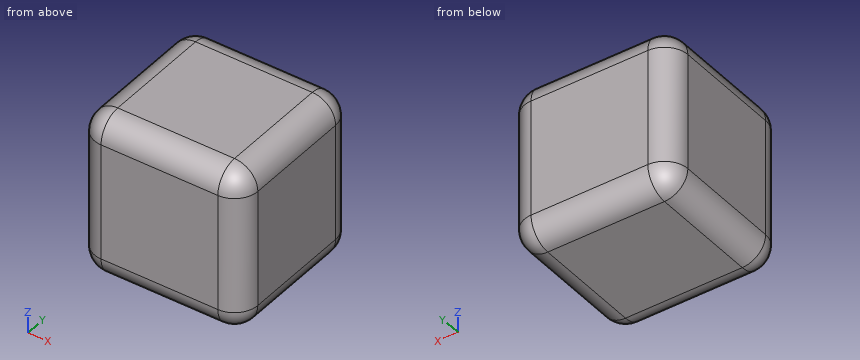
Autodesk Inventor part; units mm, degrees
ref_plane "YZ Plane" through (0, 0, 0) normal (1, 0, 0) x (0, 1, 0)
ref_plane "XZ Plane" through (0, 0, 0) normal (0, 1, 0) x (-1, 0, 0)
ref_plane "XY Plane" through (0, 0, 0) normal (0, 0, 1) x (1, 0, 0)
sketch "Эскиз1" plane through (0, 0, 0) normal (0, 1, 0) x (-1, 0, 0)
  line L0 (5.25, 5.25) -> (-5.25, 5.25)
  line L1 (-5.25, 5.25) -> (-5.25, -5.25)
  line L2 (-5.25, -5.25) -> (5.25, -5.25)
  line L3 (5.25, -5.25) -> (5.25, 5.25)
  line L4 (5.25, 0) -> (-5.25, 0) construction
  line L5 (0, 5.25) -> (0, -5.25) construction
  line L6 (3.5, -3.5) -> (-3.5, -3.5)
  line L7 (-3.5, -3.5) -> (-3.5, 3.5)
  line L8 (-3.5, 3.5) -> (3.5, 3.5)
  line L9 (3.5, 3.5) -> (3.5, -3.5)
  line L10 (0, -3.5) -> (0, 3.5) construction
  line L11 (3.5, 0) -> (-3.5, 0) construction
  point P0 (0, 0)
  point P1 (0, 0)
  point P2 (0, 0)
  dimension "d0" = 10.5
  dimension "d1" = 10.5
  dimension "d4" = 7
  dimension "d5" = 7
extrude "Выдавливание1" add sketch "Эскиз1" along normal blind 10 contours L3 L2 L1 L0 | L6 L7 L8 L9
ref_plane "РабПлоскость1" through (0, 2, 0) normal (0, -1, 0) x (1, 0, 0)
extrude "Выдавливание2" cut sketch "Эскиз1" along normal blind 6 from surface at 2 contours L6 L7 L8 L9
fillet "Сопряжение1" radius 1.5 12 edges at (-5.25, 5, -5.25) (-5.25, 0, 0) (0, 0, -5.25) (-5.25, 5, 5.25) (-5.25, 10, 0) (0, 10, -5.25) (0, 10, 5.25) (5.25, 0, 0) (5.25, 5, 5.25) (5.25, 10, 0) (5.25, 5, -5.25) (0, 0, 5.25)
properties part number "cube"
Build history of the part. All positions in model axes, mm. Coordinates: 2 decimals unless noted, no trailing zeros. Order: outer loops, then holes, each group sorted by start corner. A loop starts at its lowest first (then second) coordinate and runs counter-clockwise, first axis right, second up. Notation, with made-up numbers: (21.5, 79.25) -> (43.5, 79.25) arc R20 ccw to (43.5, 89.25) -> close; hole circle Ø5 at (-9, 55). An arc over 180 degrees is marked (long way). Answer in a Markdown table with one row per item. Add a question column.
Q1. Band-saw the part on B-B, the plane z = -0.5. List the corners of the cut face in (x, y).
Q2. Band-saw the part on C-C, the plane x = 4. List the corners of the cut face in (y, z), then the cut area to 3 significant figures.
Q3. Wall check: line 1 along X through (y, z) = (6.5, 3); line 2 along Y through (x, z) = (-3.25, -1). Give the ranges that are in metal, low to high. Write a range as [from, to].
Q4. Band-saw the part on D-D, the plane z = 4.5. List the corners of the cut face in (x, y), then the cut area to 3 significant figures.
Q5. Band-saw the part on A-A, the plane y = 7.25. List the corners of the cut face in (x, z).
Answers follow:
| question | item | result |
|---|---|---|
| 1 | outline | (-5.25, 1.5) arc R1.5 ccw to (-3.75, 0) -> (3.75, 0) arc R1.5 ccw to (5.25, 1.5) -> (5.25, 8.5) arc R1.5 ccw to (3.75, 10) -> (-3.75, 10) arc R1.5 ccw to (-5.25, 8.5) -> close; hole (-3.5, 2) -> (3.5, 2) -> (3.5, 8) -> (-3.5, 8) -> close |
| 2 | outline | (0.02, -3.75) arc R1.48 ccw to (1.5, -5.23) -> (8.5, -5.23) arc R1.48 ccw to (9.98, -3.75) -> (9.98, 3.75) arc R1.48 ccw to (8.5, 5.23) -> (1.5, 5.23) arc R1.48 ccw to (0.02, 3.75) -> close |
| 2 | area | 102 mm^2 |
| 3 | line 1 | [-5.25, -3.5], [3.5, 5.25] |
| 3 | line 2 | [0, 2], [8, 10] |
| 4 | outline | (-5.05, 1.5) arc R1.3 ccw to (-3.75, 0.2) -> (3.75, 0.2) arc R1.3 ccw to (5.05, 1.5) -> (5.05, 8.5) arc R1.3 ccw to (3.75, 9.8) -> (-3.75, 9.8) arc R1.3 ccw to (-5.05, 8.5) -> close |
| 4 | area | 95.5 mm^2 |
| 5 | outline | (-5.25, -3.75) arc R1.5 ccw to (-3.75, -5.25) -> (3.75, -5.25) arc R1.5 ccw to (5.25, -3.75) -> (5.25, 3.75) arc R1.5 ccw to (3.75, 5.25) -> (-3.75, 5.25) arc R1.5 ccw to (-5.25, 3.75) -> close; hole (-3.5, -3.5) -> (3.5, -3.5) -> (3.5, 3.5) -> (-3.5, 3.5) -> close |
